```python
from build123d import *

# Parameters (mm, degrees)
SKETCH1_W              = 36
SKETCH1_H              = 40
BASE_FLANGE1_DEPTH     = 0.7
SKETCHED_BEND1_DEPTH   = 40
SKETCHED_BEND1_2_DEPTH = 40


# Read off the part's stored shape, not the designer's step: Sketched Bend1
# Sheet-metal steps are written as plain solids
with BuildPart() as part:
    # Sketch1 → Base-Flange1 (new body)
    with BuildSketch(Plane.XY):
        with Locations((18, 20)):
            Rectangle(SKETCH1_W, SKETCH1_H)
    extrude(amount=-BASE_FLANGE1_DEPTH)

    # Sketched Bend1 outline → Sketched Bend1 (cut)
    with BuildSketch(Plane(origin=(0, 0, 0), x_dir=(1, 0, 0), z_dir=(0, 1, 0))):
        with BuildLine():
            ThreePointArc((17.146586356, 0.7), (17.855677324, 0.512803682), (18.379971941, 0))
            Line((18.379971941, 0), (36, 0))
            Line((36, 0), (36, 0.7))
            Line((36, 0.7), (17.146586356, 0.7))
        make_face()
    extrude(amount=SKETCHED_BEND1_DEPTH, mode=Mode.SUBTRACT)

    # Sketched Bend1 2 outline → Sketched Bend1 2 (add)
    with BuildSketch(Plane(origin=(0, 0, 0), x_dir=(1, 0, 0), z_dir=(0, 1, 0))):
        with BuildLine():
            Line((17.883186356, -0.7366), (17.883186356, -17.883186356))
            Line((17.883186356, -17.883186356), (18.583186356, -17.883186356))
            Line((18.583186356, -17.883186356), (18.583186356, -0.7366))
            ThreePointArc((18.583186356, -0.7366), (18.531451203, -0.354541216), (18.379971941, 0))
            Line((18.379971941, 0), (17.146586356, 0))
            ThreePointArc((17.146586356, 0), (17.667441211, -0.215745145), (17.883186356, -0.7366))
        make_face()
    extrude(amount=SKETCHED_BEND1_2_DEPTH)


solid = part.part
```
The listing builds one solid part. Answer for the finished solid, in the listing's coordinates (mm). A direction names the side the tool comes from. Give positions to 0.01 mm unless a question says otherwise; leave off trailing zeros. Order: outer loops, then holes, each group sorted by start corner. A loop starts at its lowest first (then second) coordinate and runs counter-clockwise, first axis right, second up. Notation, with made-up numbers: (14.5, 13) - (25.5, 13) arc R31 ccw to (25.5, 41) - close; hole circle Ø4 at (87, 27.25). An arc over 180 degrees is marked (long way). Use one line per item in the form item = value. Start each with the question number.
(1) A cutting plane is placed at B-B, the plane x = 13.5. Write down the section's boundary in (y, z), then the cut area to 3 significant figures.
(2) For faces 1 (the flat face through (8, 20, 0)), 2 (the flat face through (18.583, 20, 9)), determine the directions among +Z, -Z, +X, -X, +Y, -Y from which every point of the face is accessible in a straight line to the end or side of a thin tool.
(3) Flat-ended cylindrical pins translate along their axes: pin 1 Ø8.5 at (x, y) = (12.5, 22) entering from +Z; pin 2 Ø8.5 at (y, z) = (20.5, 13) entering from -X; pin 3 Ø8 at (x, z) = (6.5, 6.5) entering from -Y. Find the tip coordinate at first contact, or state that the pin passes through.
(4) A cutting plane is placed at C-C, the plane z = 10. Write down the section's boundary in (x, y).
(5) A cutting plane is placed at A-A, the plane y = 17.5. Write down the section's boundary in (x, z).
(6) Consider line 1 (Z direction, x = 8.5, y = 12); line 2 (X direction, y = 34, z = 7.25). Determine where each line is inside the solid, lowest interval first. Write a range as from..to.
Ans:
q1.outline = (0, -0.7) - (40, -0.7) - (40, 0) - (0, 0) - close
q1.area = 28.0 mm^2
q2.face_1 = +Z, -X, +Y, -Y
q2.face_2 = +Z, -Z, +X, +Y, -Y
q3.pin_1 = 0
q3.pin_2 = 17.88
q3.pin_3 = through
q4.outline = (17.88, 0) - (18.58, 0) - (18.58, 40) - (17.88, 40) - close
q5.outline = (0, -0.7) - (17.15, -0.7) arc R1.44 ccw to (18.58, 0.74) - (18.58, 17.88) - (17.88, 17.88) - (17.88, 0.74) arc R0.74 cw to (17.15, 0) - (0, 0) - close
q6.line_1 = -0.7..0
q6.line_2 = 17.88..18.58
